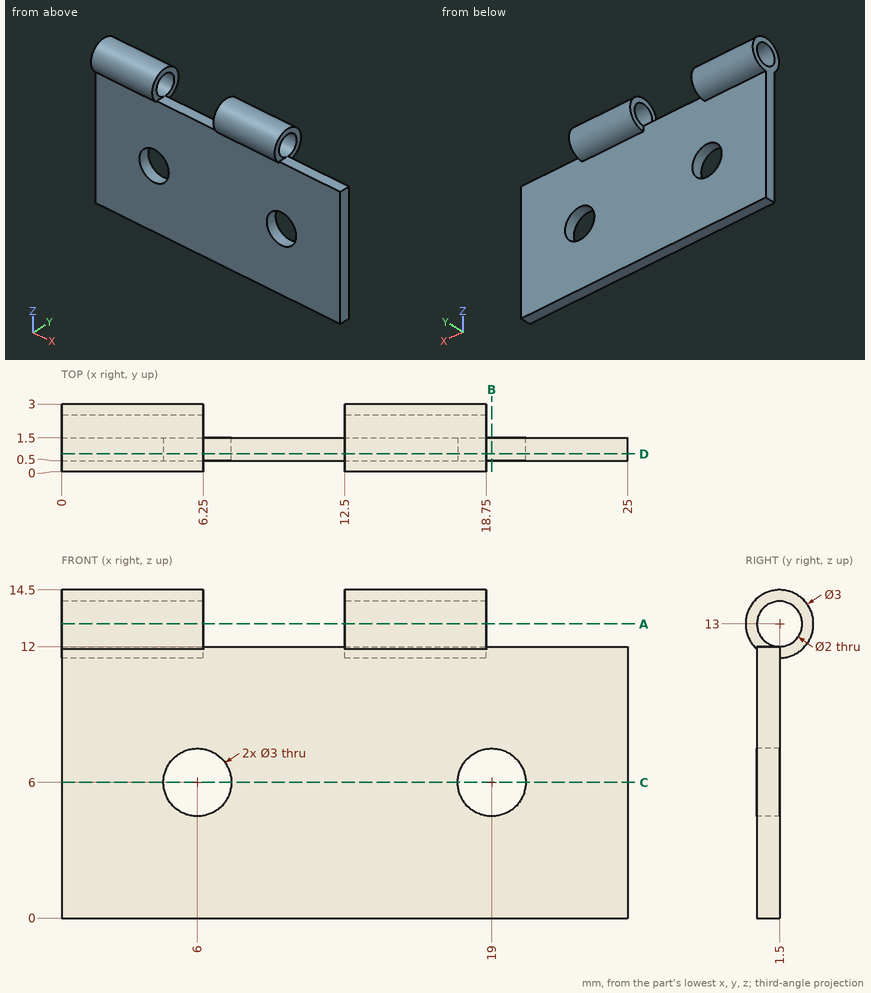
Answer from the drawing. Dimensions are ordinates in mm from the lowest x, y and z of the part. Round coordinates to 2 decimals unless told otherwise and drop trailing zeros. Write each loop counter-clockwise with the first axis right and the second up, starting at its lowest first coordinate (ties: lowest second). Pieces come first, ordered by that corner, then holes. Notation, with made-up numbers: (-28, -30) -> (-10, -30) arc R22 cw to (-10, -7) -> close; hole circle Ø6 at (83.25, 55.25). An arc over 180 degrees is marked (long way). Answer in a Markdown table with one row per item. Add a question column.
1) Find section D-D, the plane y = 0.8. Determine the outline of the cut face in (x, z), and give its area (3 significant figures).
2) Find section A-A, the plane z = 13. Determine the outline of the cut face in (x, y).
3) Find section C-C, the plane z = 6. Determine the outline of the cut face in (x, y).
4) Find section B-B, the plane x = 19. Determine the outline of the cut face in (y, z).
5) Consider line 1 (X direction, y = 1.15, z = 6); line 2 (Y direction, x = 17.25, z = 13); line 3 (X direction, y = 0.55, z = 5). Determine where each line is inside the solid, lowest interval first.
6) Given P1, Ø3, axis at x = 18.5, z = 10.5, coming from the +Y side; P2, Ø1.5, axis at x = 8, y = 0.5, coming from the +Z side; P3, Ø3.5, axis at x = 11, z = 4, coming from the -Y side, each flat-ended and moving along its own axis, determine where each tip first touches the part or whether it passes through.
Findings below:
| question | item | result |
|---|---|---|
| 1 | outline | (0, 0) -> (25, 0) -> (25, 12) -> (18.75, 12) -> (18.75, 12.29) -> (12.5, 12.29) -> (12.5, 12) -> (6.25, 12) -> (6.25, 12.29) -> (0, 12.29) -> close; (0, 13.71) -> (6.25, 13.71) -> (6.25, 14.33) -> (0, 14.33) -> close; (12.5, 13.71) -> (18.75, 13.71) -> (18.75, 14.33) -> (12.5, 14.33) -> close; hole circle Ø3 at (6, 6); hole circle Ø3 at (19, 6) |
| 1 | area | 297 mm² |
| 2 | outline | (0, 0) -> (6.25, 0) -> (6.25, 0.5) -> (0, 0.5) -> close; (0, 2.5) -> (6.25, 2.5) -> (6.25, 3) -> (0, 3) -> close; (12.5, 0) -> (18.75, 0) -> (18.75, 0.5) -> (12.5, 0.5) -> close; (12.5, 2.5) -> (18.75, 2.5) -> (18.75, 3) -> (12.5, 3) -> close |
| 3 | outline | (0, 0.5) -> (4.5, 0.5) -> (4.5, 1.5) -> (0, 1.5) -> close; (7.5, 0.5) -> (17.5, 0.5) -> (17.5, 1.5) -> (7.5, 1.5) -> close; (20.5, 0.5) -> (25, 0.5) -> (25, 1.5) -> (20.5, 1.5) -> close |
| 4 | outline | (0.5, 0) -> (1.5, 0) -> (1.5, 4.5) -> (0.5, 4.5) -> close; (0.5, 7.5) -> (1.5, 7.5) -> (1.5, 12) -> (0.5, 12) -> close |
| 5 | line 1 | 0 to 4.5, 7.5 to 17.5, 20.5 to 25 |
| 5 | line 2 | 0 to 0.5, 2.5 to 3 |
| 5 | line 3 | 0 to 4.88, 7.12 to 17.88, 20.12 to 25 |
| 6 | P1 | y = 2.62 |
| 6 | P2 | z = 12 |
| 6 | P3 | y = 0.5 |
